Read the model definition and answer for the solid it produces. Units are mm, in the model's axes. A direction names the side the tool comes from. Coordinates: 2 decimals unless noted, no trailing zeros. Loops run counter-clockwise (first coordinate to the right, second up) from the corner with the lowest first, then second, coordinate; pieces in that order, holes last.
Autodesk Inventor part; units mm, degrees
sketch "Sketch1" plane through (0, 0, 0) normal (0, 0, 1) x (1, 0, 0)
  line L0 (0, 2.8582) -> (0, -2.8582) construction
  line L1 (-5.7775, 0) -> (5.7775, 0) construction
  circle A0 centre (0, 0) radius 6
  circle A1 centre (0, 0) radius 3.1
  dimension "d0" = 12
  dimension "d1" = 6.2
extrude "Extrusion1" add sketch "Sketch1" along normal blind 16.5
sketch "Sketch2" plane through (0, 0, 16.5) normal (0, 0, 1) x (1, 0, 0)
  circle A0 centre (0, 0) radius 4.5
  circle A1 centre (0, 0) radius 9
  dimension "d4" = 9
  dimension "d5" = 18
extrude "Extrusion2" add sketch "Sketch2" against normal blind 2
fillet "Fillet1" radius 2 1 edges at (-6, 0, 14.5)
properties part number "Hoes" material "S235"
Q1. Straight lines are drawn through the part: probe 1 along Y at (x, z) = (0, 9.25); probe 2 along Z at (x, y) = (4.25, -7.5); probe 3 along Y at (x, z) = (0.75, 11.25). For each, find the intervals that lie inside material, in ascending order.
Findings below:
probe 1: y = -6 to -3.1, 3.1 to 6
probe 2: z = 14.5 to 16.5
probe 3: y = -5.95 to -3.01, 3.01 to 5.95
Q2. Flat-ended cylindrical pins translate along their axes: pin 1 Ø5.5 at (x, y) = (-1.5, 4) entering from -Z; pin 2 Ø4 at (x, z) = (1.5, 8) entering from -Y; pin 3 Ø5.5 at (x, y) = (0, 0) entering from +Z; pin 4 Ø1 at (y, z) = (-2.5, 3) entering from -X. Find the tip coordinate at first contact, or state that the pin passes through.
Findings below:
pin 1: stops at z = 0
pin 2: stops at y = -6
pin 3: passes through
pin 4: stops at x = -5.66
Q3. A cutting plane is placed at D-D (z = 7.5). Give the vertices of the cut face in (x, y).
Findings below:
outline: circle Ø12 at (0, 0); hole circle Ø6.2 at (0, 0)
Q4. A cutting plane is placed at A-A (x = 0). Give the vertices of the cut face in (y, z), then the cut area to 3 significant figures.
Findings below:
outline: (-9, 14.5) - (-8, 14.5) arc R2 cw to (-6, 12.5) - (-6, 0) - (-3.1, 0) - (-3.1, 16.5) - (-9, 16.5) - close; (3.1, 0) - (6, 0) - (6, 12.5) arc R2 cw to (8, 14.5) - (9, 14.5) - (9, 16.5) - (3.1, 16.5) - close
area: 109 mm2
Q5. Determine the mould class of faces 3 (the face through (0, -4, 16.5)), 4 (the face through (1.43, 2.75, 8.13)), 5 (the face through (-1.172, 8.923, 15.514)) for opening direction X: +X half, -X half, draft (parallel to the pull), parting line (faces both ways), or undercut.
Findings below:
face 3: draft
face 4: undercut
face 5: parting line
Q6. A cutting plane is placed at C-C (z = 15). Give the vertices of the cut face in (x, y), then the cut area to 3 significant figures.
Findings below:
outline: circle Ø18 at (0, 0); hole circle Ø6.2 at (0, 0)
area: 224 mm2
Q7. Which of the six approach directions +Z, -Z, +X, -X, +Y, -Y give full straight-line access (tool end or side, diameter ignored) to faces 1 (the face through (-6, 0, 6)), 2 (the face through (3, -3, 0))?
Findings below:
face 1: -Z
face 2: -Z, +X, -X, +Y, -Y
